Can you work these out from the model? Positions are in its coordinate system, mm. A direction names the side the tool comes from. Coordinates: 2 decimals unless noted, no trailing zeros. Order: outer loops, then holes, each group sorted by start corner. A loop starts at its lowest first (then second) coordinate and runs counter-clockwise, first axis right, second up. Notation, with made-up numbers: (-26.5, 9.25) -> (3.5, 9.25) arc R24 ccw to (3.5, 24.25) -> close; hole circle Ø3 at (-12, 81.25). An arc over 180 degrees is marked (long way). Answer as a JSON object with one key per item and string values. Group by question number.
(1) I need wall thicknesses on line 1 (Z direction, x = 132.5, y = 1); line 2 (X direction, y = 2.9, z = -32.5) (3 decimals); line 3 (X direction, y = 1.3, z = 30.25). Which ranges of each line are inside material? Lowest first, please.
(2) Which directions (+Z, -Z, +X, -X, +Y, -Y) give clear straight access to the entire face, cutting with the end or side of a thin tool? Please do faces 5 (the flat face through (0, 2, 20)), 6 (the flat face through (184.067, 1.972, 5.783)), 7 (the flat face through (109, 2, -22)).
(3) I want a section at B-B, the plane y = 0.6. State how many separate pieces and enclosed holes the cut face has, plus the area to 3 significant figures.
(4) I want a section at A-A, the plane z = 15.5. List the corners of the cut face in (x, y) for me, plus the area to 3 significant figures.
(5) If we mould it in two halves opening along X, with no side actions, what happens to faces 1 (the flat face through (87, 4, -12)), 2 (the flat face through (103.87, 1.97, -23.49)), 3 (the flat face through (66.13, 1.97, -23.49)), 4 (the flat face through (167, 2, -42))? For each: pulls with the +X half, pulls with the -X half, needs draft (parallel to the pull), parting line crosses it, or undercut.
(6) I want a section at C-C, the plane x = 3.5. List the corners of the cut face in (y, z) for me.
(7) For pin 1 (1.2 mm diameter, centred on y = 2, z = -19.5, fed in from -X); pin 2 (2 mm diameter, centred on y = 2, z = -27, fed in from +X); pin 3 (1.9 mm diameter, centred on x = 195.25, z = 30.25, fed in from +Y); pin 4 (2 mm diameter, centred on x = 72.5, y = 2.5, fed in from +Z), each with a flat end and sliding along its axis, tell me the tip position at first contact or that it passes through.
from build123d import *

# Parameters (mm, degrees)
SKETCH_1_W          = 170
SKETCH_1_H          = 45
SKETCH_1_R          = 2
SKETCH_1_R_2        = 2.1
EXTRUDE_1_DEPTH     = 4
EXTRUDE_2_DEPTH     = 4
CUT_EXTRUDE_1_DEPTH = 4
CUT_EXTRUDE_2_DEPTH = 4
FILLET_1_R          = 2
SKETCH_6_R          = 1.6
CUT_EXTRUDE_3_DEPTH = 50


with BuildPart() as part:
    # 草图1 → 凸台-拉伸1 (new body)
    with BuildSketch(Plane(origin=(0, 0, 0), x_dir=(1, 0, 0), z_dir=(0, 1, 0))):
        with Locations((85, 22.5)):
            Rectangle(SKETCH_1_W, SKETCH_1_H)
        with Locations(Location((10, 35, 0), (0, 0, 270))):
            Circle(SKETCH_1_R, mode=Mode.SUBTRACT)
        with Locations(Location((10, 10, 0), (0, 0, 270))):
            Circle(SKETCH_1_R, mode=Mode.SUBTRACT)
        with Locations(Location((160, 10, 0), (0, 0, 270))):
            Circle(SKETCH_1_R, mode=Mode.SUBTRACT)
        with Locations(Location((160, 35, 0), (0, 0, 270))):
            Circle(SKETCH_1_R, mode=Mode.SUBTRACT)
        with Locations(Location((37.5, 35, 0), (0, 0, 270))):
            Circle(SKETCH_1_R_2, mode=Mode.SUBTRACT)
        with Locations(Location((37.5, 10, 0), (0, 0, 270))):
            Circle(SKETCH_1_R_2, mode=Mode.SUBTRACT)
        with Locations(Location((132.5, 10, 0), (0, 0, 270))):
            Circle(SKETCH_1_R_2, mode=Mode.SUBTRACT)
        with Locations(Location((132.5, 35, 0), (0, 0, 270))):
            Circle(SKETCH_1_R_2, mode=Mode.SUBTRACT)
    extrude(amount=EXTRUDE_1_DEPTH)

    # 草图2 → 凸台-拉伸2 (add)
    with BuildSketch(Plane(origin=(0, 0, 0), x_dir=(1, 0, 0), z_dir=(0, 1, 0))):
        Polygon((170, 8.284271247), (198.534271247, -20.25), (220.25, -20.25), (220.25, -40.25), (190.25, -40.25), (150, 0), (170, 0), align=None)
        Polygon((-50.25, -40.25), (-20.25, -40.25), (20, 0), (0, 0), (0, 8.284271247), (-28.534271247, -20.25), (-50.25, -20.25), align=None)
    extrude(amount=EXTRUDE_2_DEPTH)

    # 草图4 → 切除-拉伸1 (cut)
    with BuildSketch(Plane(origin=(0, 4, 0), x_dir=(1, 0, 0), z_dir=(0, 1, 0))):
        Polygon((0, 38.909451479), (6, 45), (0, 45), align=None)
        Polygon((170, 39), (164, 45), (170, 45), align=None)
    extrude(amount=-CUT_EXTRUDE_1_DEPTH, mode=Mode.SUBTRACT)

    # 草图5 → 切除-拉伸2 (cut)
    with BuildSketch(Plane.XZ):
        Polygon((47.5, -5), (47.5, -40), (73.75, -5), align=None)
        Polygon((53.75, -40), (80, -5), (80, -40), align=None)
        Polygon((90, -5), (90, -40), (116.25, -40), align=None)
        Polygon((96.25, -5), (122.5, -5), (122.5, -40), align=None)
    extrude(amount=-CUT_EXTRUDE_2_DEPTH, mode=Mode.SUBTRACT)

    # 圆角1
    fillet_1_edges = [part.edges().sort_by_distance(p)[0] for p in [
        (80, 2, -5),
        (53.75, 2, -40),
        (80, 2, -40),
        (90, 2, -40),
        (116.25, 2, -40),
        (90, 2, -5),
        (122.5, 2, -5),
        (96.25, 2, -5),
        (122.5, 2, -40),
        (47.5, 2, -40),
        (73.75, 2, -5),
        (47.5, 2, -5),
    ]]
    fillet(fillet_1_edges, radius=FILLET_1_R)

    # 草图6 → 切除-拉伸3 (cut)
    with BuildSketch(Plane.XZ):
        with Locations(Location((-45.25, 30.25, 0), (0, 0, 270))):
            Circle(SKETCH_6_R)
        with Locations(Location((-25.25, 30.25, 0), (0, 0, 270))):
            Circle(SKETCH_6_R)
        with Locations(Location((195.25, 30.25, 0), (0, 0, 90))):
            Circle(SKETCH_6_R)
        with Locations(Location((215.25, 30.25, 0), (0, 0, 90))):
            Circle(SKETCH_6_R)
    extrude(amount=-CUT_EXTRUDE_3_DEPTH, mode=Mode.SUBTRACT)


solid = part.part
Computed values:
{
 "1": {"line 1": "z = -45 to -37.1, -32.9 to -12.1, -7.9 to 0", "line 2": "x = 0 to 47.5, 53.125 to 59.375, 80 to 90, 110.625 to 116.875, 122.5 to 170", "line 3": "x = -50.25 to -46.85, -43.65 to -26.85, -23.65 to -10.25, 180.25 to 193.65, 196.85 to 213.65, 216.85 to 220.25"},
 "2": {"face 5": "+Z, +Y, -Y", "face 6": "-Z, +X, +Y, -Y", "face 7": "+Y, -Y"},
 "3": {"separate pieces": "1", "enclosed holes": "16", "area": "8,500 mm2"},
 "4": {"outline": "(-23.78, 0) -> (4.5, 0) -> (4.5, 4) -> (-23.78, 4) -> close; (165.5, 0) -> (193.78, 0) -> (193.78, 4) -> (165.5, 4) -> close", "area": "226 mm2"},
 "5": {"face 1": "needs draft", "face 2": "undercut", "face 3": "undercut", "face 4": "pulls with the +X half"},
 "6": {"outline": "(0, -42.46) -> (4, -42.46) -> (4, 16.5) -> (0, 16.5) -> close"},
 "7": {"pin 1": "stops at x = 0", "pin 2": "stops at x = 170", "pin 3": "passes through", "pin 4": "stops at z = 0"}
}
